from build123d import *

# Parameters (mm, degrees)
SKETCH1_W          = 12.5
SKETCH1_H          = 12.5
CUVETTE_BODY_DEPTH = 45
SAMPLE_SPACE_START = 45
SKETCH2_W          = 10
SKETCH2_H          = 10
SAMPLE_SPACE_DEPTH = 43.75


with BuildPart() as part:
    # Sketch1 → Cuvette_Body (new body)
    with BuildSketch(Plane(origin=(0, 0, 0), x_dir=(1, 0, 0), z_dir=(0, 1, 0))):
        Rectangle(SKETCH1_W, SKETCH1_H)
    extrude(amount=CUVETTE_BODY_DEPTH)

    # Sketch2 → Sample_Space (cut)
    with BuildSketch(Plane(origin=(0, 0, 0), x_dir=(1, 0, 0), z_dir=(0, 1, 0)).offset(SAMPLE_SPACE_START)):
        Rectangle(SKETCH2_W, SKETCH2_H)
    extrude(amount=-SAMPLE_SPACE_DEPTH, mode=Mode.SUBTRACT)


solid = part.part
Verification items for the finished model (mm, model axes). A direction names the side the tool comes from. Coordinates: 2 decimals unless noted, no trailing zeros. Loops run counter-clockwise (first coordinate to the right, second up) from the corner with the lowest first, then second, coordinate; pieces in that order, holes last. Notation, with made-up numbers: (-13, 6) -> (39, 6) arc R19 cw to (39, 36) -> close; hole circle Ø1 at (-13, 80.25). An arc over 180 degrees is marked (long way). Write each question's results on one line, items separated by ' | '.
Item 1: Section check A-A, the plane y = 23. Enter the section's corners in (x, z).
Found:
outline: (-6.25, -6.25) -> (6.25, -6.25) -> (6.25, 6.25) -> (-6.25, 6.25) -> close; hole (-5, -5) -> (5, -5) -> (5, 5) -> (-5, 5) -> close
Item 2: Section check B-B, the plane x = 4. Enter the section's corners in (y, z), plus the area to 3 significant figures.
Found:
outline: (0, -6.25) -> (45, -6.25) -> (45, -5) -> (1.25, -5) -> (1.25, 5) -> (45, 5) -> (45, 6.25) -> (0, 6.25) -> close | area: 125 mm2
Item 3: Mould release check, pull along Z, two halves, no side actions. Record for faces 1 (the face through (0, 22, -6.25)), 2 (the face through (0, 22, 6.25)), 3 (the face through (0, 23, -5)), 4 (the face through (0, 0, 0)): +Z half, -Z half, draft (parallel to the pull), parting line (faces both ways), or undercut.
Found:
face 1: -Z half | face 2: +Z half | face 3: undercut | face 4: draft
Item 4: Section check C-C, the plane z = 0.25. Enter the section's corners in (x, y), plus the area to 3 significant figures.
Found:
outline: (-6.25, 0) -> (6.25, 0) -> (6.25, 45) -> (5, 45) -> (5, 1.25) -> (-5, 1.25) -> (-5, 45) -> (-6.25, 45) -> close | area: 125 mm2
Item 5: Gauge pin test, flat ends, axial feed: pin 1 (6 mm diameter, centred on x = 4.5, z = 5, fed in from -Y); pin 2 (3 mm diameter, centred on x = -2, z = 2, fed in from +Y). Record the tip position at first contact, or that the pin passes through.
Found:
pin 1: stops at y = 0 | pin 2: stops at y = 1.25
Item 6: Tool access check on faces 5 (the face through (-6.25, 22, 0)), 6 (the face through (0, 23, 5)). Record the directions out of +Z, -Z, +X, -X, +Y, -Y that give a thin tool (end or side, any length) a straight path to the whole face; none if there is none.
Found:
face 5: +Z, -Z, -X, +Y, -Y | face 6: +Y
Item 7: Material ranges on L1, parallel to Z at x = 2.5, y = 18; L2, parallel to Y at x = 2.5, z = 2.75, recorded low to high.
Found:
L1: z = -6.25 to -5, 5 to 6.25 | L2: y = 0 to 1.25
